For this review, take the finished solid that the model builds, in its own axes (mm). Give positions to 0.01 mm unless a question says otherwise; leave off trailing zeros. Order: outer loops, then holes, each group sorted by start corner. A loop starts at its lowest first (then second) coordinate and runs counter-clockwise, first axis right, second up.
Item 1: For probe 1 along Y at (x, z) = (120, 1.2); probe 2 along Y at (x, z) = (20, 1.2); probe 3 along X at (y, z) = (11.5, 0.9), list the stretches that pass through material, from the lowest coordinate up.
Item 2: Consider section B-B (x = 120). Give the boundary of the cut face in (y, z), plus the area to 3 significant figures.
Item 3: Consider section C-C (z = 0.95). Give the number of separate pieces and of enclosed holes in the cut face, plus the area to 3 significant figures.
Item 4: Consider section A-A (x = 19). Give the boundary of the cut face in (y, z).
Item 5: For P1, Ø1.7, axis at x = 143, y = 25, coming from the +Z side, flat-tipped, find the tip position at first contact; note if it passes through.
```python
from build123d import *

# Parameters (mm, degrees)
SKETCH_1_W          = 148
SKETCH_1_H          = 50
EXTRUDE_1_DEPTH     = 3
SKETCH_2_R          = 1.45
CUT_EXTRUDE_1_DEPTH = 157.246599963
SKETCH_3_W          = 15
SKETCH_3_H          = 16
CUT_EXTRUDE_2_DEPTH = 10
FILLET_1_R          = 3
FILLET_2_R          = 2.5


with BuildPart() as part:
    # 草图1 → 凸台-拉伸1 (new body)
    with BuildSketch(Plane.XY):
        with Locations((74, 25)):
            Rectangle(SKETCH_1_W, SKETCH_1_H)
    extrude(amount=EXTRUDE_1_DEPTH)

    # 草图2 → 切除-拉伸1 (cut, through all)
    with BuildSketch(Plane.XY.offset(3)):
        with Locations((5, 35)):
            Circle(SKETCH_2_R)
        with Locations((5, 25)):
            Circle(SKETCH_2_R)
        with Locations((5, 15)):
            Circle(SKETCH_2_R)
        with Locations((28, 15)):
            Circle(SKETCH_2_R)
        with Locations((28, 25)):
            Circle(SKETCH_2_R)
        with Locations((28, 35)):
            Circle(SKETCH_2_R)
        with Locations((120, 35)):
            Circle(SKETCH_2_R)
        with Locations((120, 25)):
            Circle(SKETCH_2_R)
        with Locations((120, 15)):
            Circle(SKETCH_2_R)
        with Locations((143, 15)):
            Circle(SKETCH_2_R)
        with Locations((143, 25)):
            Circle(SKETCH_2_R)
        with Locations((143, 35)):
            Circle(SKETCH_2_R)
        with Locations((41.5, 42)):
            Circle(SKETCH_2_R)
        with Locations((106.5, 42)):
            Circle(SKETCH_2_R)
        with Locations((106.5, 8)):
            Circle(SKETCH_2_R)
        with Locations((41.5, 8)):
            Circle(SKETCH_2_R)
    extrude(amount=-CUT_EXTRUDE_1_DEPTH, mode=Mode.SUBTRACT)

    # 草图3 → 切除-拉伸2 (cut)
    with BuildSketch(Plane.XY.offset(3)):
        Polygon((49, 43), (99, 43), (74, 27.111036145), align=None)
        Polygon((48.059067085, 12.326369507), (68, 25), (48.059067085, 37.673630493), (36.5, 31), (36.5, 19), align=None)
        Polygon((99.940932915, 12.326369507), (80, 25), (99.940932915, 37.673630493), (111.5, 31), (111.5, 19), align=None)
        Polygon((74, 22.888963855), (49, 7), (99, 7), align=None)
        with Locations((16.5, 36)):
            Rectangle(SKETCH_3_W, SKETCH_3_H)
        with Locations((16.5, 14)):
            Rectangle(SKETCH_3_W, SKETCH_3_H)
        with Locations((131.5, 36)):
            Rectangle(SKETCH_3_W, SKETCH_3_H)
        with Locations((131.5, 14)):
            Rectangle(SKETCH_3_W, SKETCH_3_H)
    extrude(amount=-CUT_EXTRUDE_2_DEPTH, mode=Mode.SUBTRACT)

    # 圆角1
    fillet_1_edges = [part.edges().sort_by_distance(p)[0] for p in [
        (0, 50, 1.5),
        (148, 50, 1.5),
        (148, 0, 1.5),
        (0, 0, 1.5),
    ]]
    fillet(fillet_1_edges, radius=FILLET_1_R)

    # 圆角2
    fillet_2_edges = [part.edges().sort_by_distance(p)[0] for p in [
        (9, 6, 1.5),
        (9, 22, 1.5),
        (24, 22, 1.5),
        (24, 6, 1.5),
        (74, 22.888963855, 1.5),
        (99, 7, 1.5),
        (49, 7, 1.5),
        (99.940932915, 37.673630493, 1.5),
        (111.5, 31, 1.5),
        (111.5, 19, 1.5),
        (99.940932915, 12.326369507, 1.5),
        (80, 25, 1.5),
        (36.5, 31, 1.5),
        (48.059067085, 37.673630493, 1.5),
        (68, 25, 1.5),
        (48.059067085, 12.326369507, 1.5),
        (36.5, 19, 1.5),
        (124, 28, 1.5),
        (124, 44, 1.5),
        (139, 44, 1.5),
        (139, 28, 1.5),
        (9, 28, 1.5),
        (9, 44, 1.5),
        (24, 44, 1.5),
        (24, 28, 1.5),
        (124, 6, 1.5),
        (124, 22, 1.5),
        (139, 22, 1.5),
        (139, 6, 1.5),
        (74, 27.111036145, 1.5),
        (49, 43, 1.5),
        (99, 43, 1.5),
    ]]
    fillet(fillet_2_edges, radius=FILLET_2_R)


solid = part.part
```
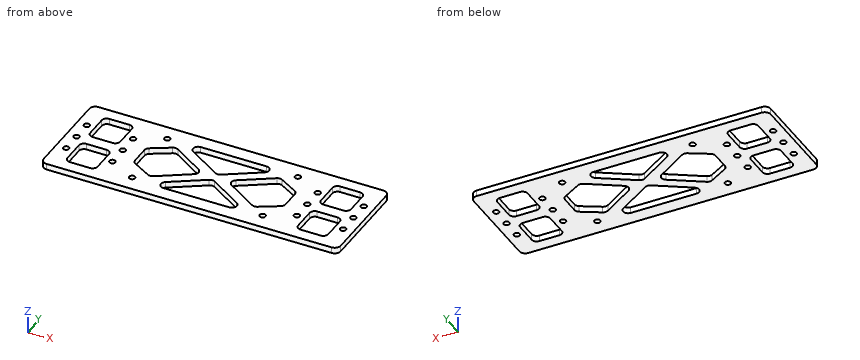
Resolved:
1. probe 1: y = 0 to 13.55, 16.45 to 23.55, 26.45 to 33.55, 36.45 to 50
1. probe 2: y = 0 to 6, 22 to 28, 44 to 50
1. probe 3: x = 0 to 9, 24 to 56.09, 91.91 to 124, 139 to 148
2. outline: (0, 0) - (13.55, 0) - (13.55, 3) - (0, 3) - close; (16.45, 0) - (23.55, 0) - (23.55, 3) - (16.45, 3) - close; (26.45, 0) - (33.55, 0) - (33.55, 3) - (26.45, 3) - close; (36.45, 0) - (50, 0) - (50, 3) - (36.45, 3) - close
2. area: 124 mm2
3. separate pieces: 1
3. enclosed holes: 24
3. area: 4,680 mm2
4. outline: (0, 0) - (6, 0) - (6, 3) - (0, 3) - close; (22, 0) - (28, 0) - (28, 3) - (22, 3) - close; (44, 0) - (50, 0) - (50, 3) - (44, 3) - close
5. P1: passes through
